The figure shows three views and two pictorial views of one solid part (mm, origin at its lowest corner). Answer the questions. Coordinates: 2 decimals unless noted, no trailing zeros. Loops run counter-clockwise (first coordinate to the right, second up) from the corner with the lowest first, then second, coordinate; pieces in that order, holes last. Notation, with made-up numbers: (44, 59.25) -> (88, 59.25) arc R24 cw to (88, 96.25) -> close; hole circle Ø1 at (71, -2). An arc over 180 degrees is marked (long way). Use a Markdown table: item, result. Add a question column.
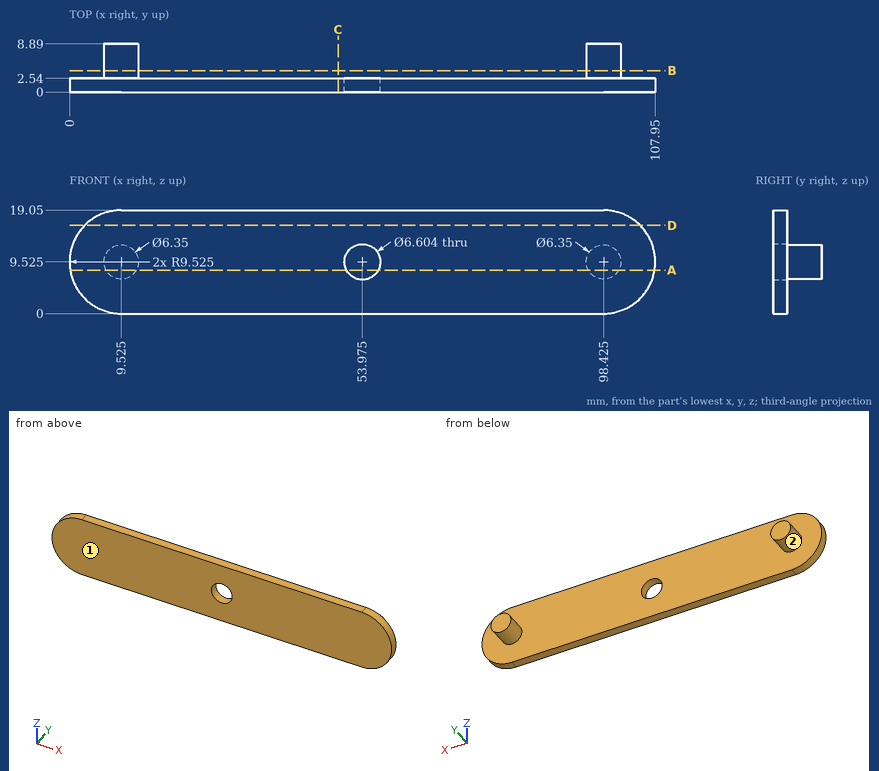
Item 1: Section D-D (z = 16.25) is taken. Determine the outline of the cut face in (x, y), then the cut area to 3 significant figures.
Item 2: Section A-A (z = 8) is taken. Determine the outline of the cut face in (x, y), then the cut area to 3 significant figures.
Item 3: Given pin 1 (1 mm diameter, centred on y = 1.5, z = 4.5, fed in from +X); pin 2 (10 mm diameter, centred on x = 36, z = 8.5, fed in from -Y); pin 3 (2 mm diameter, centred on x = 26, z = 6, fed in from +Y); pin 4 (1 mm diameter, centred on y = 2.5, z = 6, fed in from +X), each flat-ended and moving along its own axis, determine where each tip first touches the part or whether it passes through.
Item 4: For a pull along X with two mould halves and no side action, classify the marked faces 1 and 2 as +X half, -X half, draft (parallel to the pull), parting line (faces both ways), or undercut.
Item 5: Find the intervals of material crossed by probe 1 along Y at (x, z) = (102.5, 7); probe 2 along X at (y, z) = (8.25, 11); probe 3 along Z at (x, y) = (55.5, 1), in increasing order.
Item 6: Section C-C (x = 49.5) is taken. Determine the outline of the cut face in (y, z).
Item 7: Section B-B (y = 4) is taken. Determine the outline of the cut face in (x, z) (3 decimals), then the cut area to 3 significant figures.
Output:
| question | item | result |
|---|---|---|
| 1 | outline | (2.78, 0) -> (105.17, 0) -> (105.17, 2.54) -> (2.78, 2.54) -> close |
| 1 | area | 260 mm2 |
| 2 | outline | (0.12, 0) -> (51.05, 0) -> (51.05, 2.54) -> (12.31, 2.54) -> (12.31, 8.89) -> (6.74, 8.89) -> (6.74, 2.54) -> (0.12, 2.54) -> close; (56.9, 0) -> (107.83, 0) -> (107.83, 2.54) -> (101.21, 2.54) -> (101.21, 8.89) -> (95.64, 8.89) -> (95.64, 2.54) -> (56.9, 2.54) -> close |
| 2 | area | 329 mm2 |
| 3 | pin 1 | stops at x = 106.81 |
| 3 | pin 2 | stops at y = 0 |
| 3 | pin 3 | stops at y = 2.54 |
| 3 | pin 4 | stops at x = 107.46 |
| 4 | face 1 | draft |
| 4 | face 2 | undercut |
| 5 | probe 1 | y = 0 to 2.54 |
| 5 | probe 2 | x = 6.71 to 12.34, 95.61 to 101.24 |
| 5 | probe 3 | z = 0 to 6.6, 12.45 to 19.05 |
| 6 | outline | (0, 0) -> (2.54, 0) -> (2.54, 19.05) -> (0, 19.05) -> close |
| 7 | outline | circle Ø6.35 at (9.525, 9.525); circle Ø6.35 at (98.425, 9.525) |
| 7 | area | 63.3 mm2 |
